Autodesk Inventor part; units mm, degrees
ref_plane "YZ Plane" through (0, 0, 0) normal (1, 0, 0) x (0, 1, 0)
ref_plane "XZ Plane" through (0, 0, 0) normal (0, 1, 0) x (-1, 0, 0)
ref_plane "XY Plane" through (0, 0, 0) normal (0, 0, 1) x (1, 0, 0)
sketch "Sketch1" plane through (0, 0, 0) normal (0, 1, 0) x (-1, 0, 0)
  line L0 (0, 0) -> (36, 0)
  line L1 (36, 0) -> (36, 28)
  line L2 (0, 28) -> (0, 0)
  arc A0 (36, 28) -> (0, 28) centre (18, 28) ccw
  circle A1 centre (18, 28) radius 8
  dimension "d0" = 36
  dimension "d1" = 28
  dimension "d2" = 16
extrude "Extrusion1" add sketch "Sketch1" along normal blind 8
sketch "Sketch2" plane through (0, 0, 0) normal (0, 0, -1) x (-1, 0, 0)
  line L0 (36, 8) -> (0, 8)
  line L1 (36, 8) -> (26, 8)
  line L2 (26, 8) -> (26, 40)
  line L3 (26, 40) -> (36, 40)
  line L4 (36, 40) -> (36, 8)
  line L5 (26, 40) -> (0, 8)
  point P0 (0, 0)
  dimension "d5" = 10
  dimension "d6" = 32
mirror "Mirror1" about plane through (0, 0, 0) normal (0, 0, 1) of "Extrusion1"
extrude "Extrusion2" add sketch "Sketch2" along normal mid plane 12 contours L0 L5 L2
extrude "Extrusion3" add sketch "Sketch2" along normal mid plane 40 contours L0 L2 L3 L4
sketch "Sketch3" plane through (-36, 40, -20) normal (0, 1, 0) x (1, 0, 0)
  line L0 (0, 8) -> (0, -48)
  circle A0 centre (-32, -20) radius 10
  circle A1 centre (-32, -20) radius 15
  line L1 (0, -48) -> (0, -40)
  line L2 (0, -40) -> (-32, -35)
  line L3 (0, 0) -> (10, 0)
  line L4 (0, 0) -> (-32, -5)
  point P0 (36, -20)
  dimension "d12" = 20
  dimension "d13" = 30
extrude "Extrusion4" add sketch "Sketch3" against normal blind 10 contours L0 L2 A1 L4
extrude "Extrusion5" add sketch "Sketch3" along normal blind 10 and the other way blind 10 contours A1
Design review of the part built by this model. Coordinates are the model's own, in mm. A direction names the side the tool comes from. Coordinates: 2 decimals unless noted, no trailing zeros. Loops run counter-clockwise (first coordinate to the right, second up) from the corner with the lowest first, then second, coordinate; pieces in that order, holes last.
Q1. We need section A-A on z = 0. State the section outline as (x, y) points.
Reported:
outline: (-83, 30) - (-78, 30) - (-78, 50) - (-83, 50) - close; (-58, 30) - (-36, 30) - (-36, 0) - (0, 0) - (0, 8) - (-26, 40) - (-53, 40) - (-53, 50) - (-58, 50) - close
Q2. The part is to be moulded in two halves that separate along Z. For faces 6 (the face through (-10, 8, -26)), 7 (the face through (-18, 4, 46)), 8 (the face through (-10, 4, 28)), 9 (the face through (-31, 24, -20)), say which applies: +Z half, -Z half, draft (parallel to the pull), parting line (faces both ways), or undercut.
Reported:
face 6: draft
face 7: +Z half
face 8: undercut
face 9: -Z half
Q3. Tool access review of faces 1 (the face through (-19, 17, 6)), 2 (the face through (-31, 24, 20)), 3 (the face through (-19, 17, -6)), 4 (the face through (-82.985, 42.082, 0.66)), 5 (the face through (-55, 30, 0)): name each direction out of +Z, -Z, +X, -X, +Y, -Y from which nothing blocks a thin tool from reaching the whole face with its end or side.
Reported:
face 1: +Z, +X, +Y
face 2: +Z, +X, -X, +Y
face 3: -Z, +X, +Y
face 4: +Y
face 5: +Z, -Z, -X, -Y
Q4. For pin 1 (9.5 mm diameter, centred on x = -18, z = 28, fed in from -Y); pin 2 (5 mm diameter, centred on y = 21.5, z = -20.5, fed in from +X); pin 3 (11 mm diameter, centred on x = -24.5, z = -33.5, fed in from +Y); pin 4 (4 mm diameter, centred on x = -73.5, z = 9.5, fed in from -Y), all flat-tipped, find the tip position at first contact; note any pin that passes through.
Reported:
pin 1: passes through
pin 2: stops at x = -26
pin 3: stops at y = 8
pin 4: stops at y = 30
Q5. We need section D-D on y = 45. State the section outline as (x, z) points, and give its area (3 significant figures).
Reported:
outline: circle Ø30 at (-68, 0); hole circle Ø20 at (-68, 0)
area: 393 mm2
Q6. To check wall thickness, follow line 1 (Z direction, x = -18, y = 5.5); line 2 (X direction, y = 44, z = 0); line 3 (X direction, y = 2.25, z = -28). State the ranges of each line that lie inside material, in increasing order.
Reported:
line 1: z = -46 to -36, -20 to 20, 36 to 46
line 2: x = -83 to -78, -58 to -53
line 3: x = -36 to -26, -10 to 0
Q7. We need section C-C on y = 12. State the section outline as (x, z) points, and give its area (3 significant figures).
Reported:
outline: (-36, -20) - (-26, -20) - (-26, -6) - (-3.25, -6) - (-3.25, 6) - (-26, 6) - (-26, 20) - (-36, 20) - close
area: 673 mm2
Q8. We need section B-B on x = -21.5. State the section outline as (y, z) points, and give its area (3 significant figures).
Reported:
outline: (0, -45.66) - (8, -45.66) - (8, -35.19) - (0, -35.19) - close; (0, -20.81) - (8, -20.81) - (8, -6) - (34.46, -6) - (34.46, 6) - (8, 6) - (8, 20.81) - (0, 20.81) - close; (0, 35.19) - (8, 35.19) - (8, 45.66) - (0, 45.66) - close
area: 818 mm2
